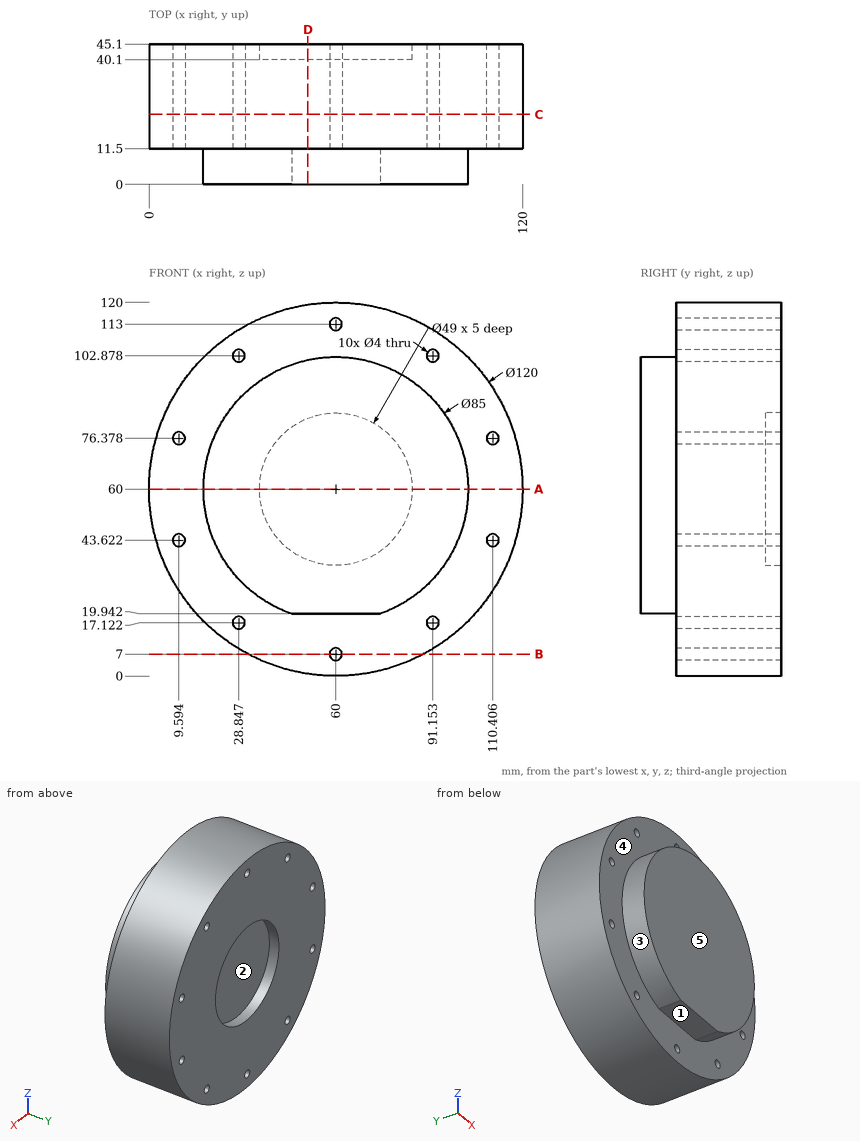
Study the drawing (mm; zero at the part's minimum x, y, z) and answer. A direction names the side the tool comes from. Round coordinates to 2 decimals unless told otherwise and drop trailing zeros. Write each loop counter-clockwise with the first axis right and the second up, starting at its lowest first coordinate (ties: lowest second). Pieces come first, ordered by that corner, then holes.
1) A cutting plane is placed at C-C on y = 22.5. Give the number of separate pieces and of enclosed holes in the cut face, and give its area (3 significant figures).
2) Consider probe 1 along X at (y, z) = (42.1, 60); probe 2 along Z at (x, y) = (60.5, 38); probe 3 along X at (y, z) = (36.5, 76). Determine where each line is inside the solid, lowest interval first.
3) Which of the six approach directions +Z, -Z, +X, -X, +Y, -Y give full straight-line access (tool end or side, diameter ignored) to the marked faces 4 and 5?
4) Determine the mould class of the marked faces 1, 2 and 3 for opening direction X: pulls with the +X half, pulls with the -X half, needs draft (parallel to the pull), parting line crosses it, or undercut.
5) Flat-ended cylindrical pins translate along their axes: P1, Ø6.5, axis at x = 110.41, z = 76.38, coming from the +Y side; P2, Ø4.5, axis at x = 9.59, z = 43.62, coming from the -Y side; P3, Ø3.5, axis at x = 91.15, z = 102.88, coming from the -Y side; P4, Ø3.5, axis at x = 60, y = 3, coming from the -Z side. Find the tip coordinate at first contact, or state that the pin passes through.
6) A cutting plane is placed at D-D on x = 51. Determine the outline of the cut face in (y, z), and give its area (3 significant figures).
7) A cutting plane is placed at A-A on z = 60. Determine the outline of the cut face in (x, y).
8) A cutting plane is placed at B-B on z = 7. Determine the outline of the cut face in (x, y) (1 decimal), and give its area (3 significant figures).
Entries:
1. separate pieces: 1
1. enclosed holes: 10
1. area: 11,200 mm2
2. probe 1: x = 0 to 35.5, 84.5 to 120
2. probe 2: z = 0 to 5.06, 8.94 to 111.06, 114.94 to 120
2. probe 3: x = 2.17 to 7.63, 11.56 to 108.44, 112.37 to 117.83
3. face 4: -Y
3. face 5: +Z, -Z, +X, -X, -Y
4. face 1: needs draft
4. face 2: undercut
4. face 3: parting line crosses it
5. P1: stops at y = 45.1
5. P2: stops at y = 11.5
5. P3: passes through
5. P4: stops at z = 19.94
6. outline: (0, 19.94) - (11.5, 19.94) - (11.5, 0.68) - (45.1, 0.68) - (45.1, 37.21) - (40.1, 37.21) - (40.1, 82.79) - (45.1, 82.79) - (45.1, 119.32) - (11.5, 119.32) - (11.5, 101.54) - (0, 101.54) - close
6. area: 4,700 mm2
7. outline: (0, 11.5) - (17.5, 11.5) - (17.5, 0) - (102.5, 0) - (102.5, 11.5) - (120, 11.5) - (120, 45.1) - (84.5, 45.1) - (84.5, 40.1) - (35.5, 40.1) - (35.5, 45.1) - (0, 45.1) - close
8. outline: (31.9, 11.5) - (58, 11.5) - (58, 45.1) - (31.9, 45.1) - close; (62, 11.5) - (88.1, 11.5) - (88.1, 45.1) - (62, 45.1) - close
8. area: 1,760 mm2
